```python
from build123d import *

# Parameters (mm, degrees)
F0_R     = 6
F0_R_2   = 4
F1_DEPTH = 1
F2_DEPTH = 7
F3_R     = 6
F3_R_2   = 4
F4_DEPTH = 2
F3_R_3   = 3.9
F3_R_4   = 0.65
F5_DEPTH = 1
F6_SIZE  = 1.5
F7_SIZE  = 0.5


with BuildPart() as f1:
    # F0 (on Top) → F1 (new body)
    with BuildSketch(Plane.XY):
        Circle(F0_R)
        Circle(F0_R_2, mode=Mode.SUBTRACT)
    extrude(amount=F1_DEPTH)

    # F0 (on Top) → F2 (join)
    with BuildSketch(Plane.XY):
        Circle(F0_R_2)
        with BuildLine():
            ThreePointArc((1.1397100223, -2.6552182762), (0.217322658, -3.2453920843), (0.0680019491, -2.1605847745))
            Line((0.0680019491, -2.1605847745), (-2.1226334177, 0.4088743166))
            ThreePointArc((-2.1226334177, 0.4088743166), (-3.1568681461, 1.1210189597), (-1.9051222763, 1.0214009718))
            Line((-1.9051222763, 1.0214009718), (1.415412254, 1.6338173044))
            ThreePointArc((1.415412254, 1.6338173044), (1.9954389417, 2.3990096505), (2.7046314686, 1.7517104579))
            ThreePointArc((2.7046314686, 1.7517104579), (2.4295432969, 1.2207291767), (1.8371203272, 1.1391838027))
            Line((1.8371203272, 1.1391838027), (0.7072211637, -2.0426916209))
            ThreePointArc((0.7072211637, -2.0426916209), (1.0206913035, -2.2803064478), (1.1397100223, -2.6552182762))
        make_face(mode=Mode.SUBTRACT)
        with BuildLine():
            Line((-2.1226334177, 0.4088743166), (0.0680019491, -2.1605847745))
            ThreePointArc((0.0680019491, -2.1605847745), (0.3718168688, -2.0159990615), (0.7072211637, -2.0426916209))
            Line((0.7072211637, -2.0426916209), (1.8371203272, 1.1391838027))
            ThreePointArc((1.8371203272, 1.1391838027), (1.5599979669, 1.3300023847), (1.415412254, 1.6338173044))
            Line((1.415412254, 1.6338173044), (-1.9051222763, 1.0214009718))
            ThreePointArc((-1.9051222763, 1.0214009718), (-1.8970422983, 0.9627003452), (-1.8943414909, 0.9035078183))
            ThreePointArc((-1.8943414909, 0.9035078183), (-1.9541676828, 0.631120454), (-2.1226334177, 0.4088743166))
        make_face()
    extrude(amount=F2_DEPTH)

    # F3 (on face) → F4 (join)
    with BuildSketch(Plane.XY.offset(7)):
        Circle(F3_R)
        Circle(F3_R_2, mode=Mode.SUBTRACT)
    extrude(amount=-F4_DEPTH)

    # F3 (on face) → F5 (cut)
    with BuildSketch(Plane.XY.offset(7)):
        Circle(F3_R_3)
        with Locations((0.4897100223, -2.6552182762)):
            Circle(F3_R_4, mode=Mode.SUBTRACT)
        with Locations((-2.5443414909, 0.9035078183)):
            Circle(F3_R_4, mode=Mode.SUBTRACT)
        with Locations((2.0546314686, 1.7517104579)):
            Circle(F3_R_4, mode=Mode.SUBTRACT)
    extrude(amount=-F5_DEPTH, mode=Mode.SUBTRACT)

    # F6
    f6_edges = [f1.edges().sort_by_distance(p)[0] for p in [
        (-6, 0, 5),
    ]]
    chamfer(f6_edges, length=F6_SIZE)

    # F7
    f7_edges = [f1.edges().sort_by_distance(p)[0] for p in [
        (-6, 0, 1),
    ]]
    chamfer(f7_edges, length=F7_SIZE)


solid = f1.part
```
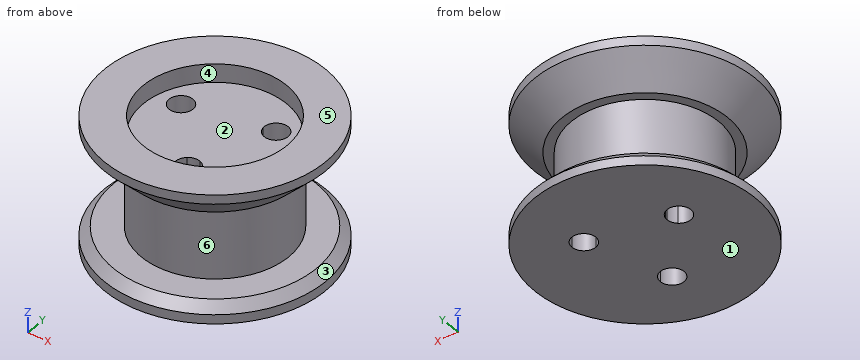
The model under review builds one solid part; all positions refer to its coordinate system, in mm. Face numbers are marked on the shaded views. A direction names the side the tool comes from. Round coordinates to 2 decimals unless told otherwise and drop trailing zeros. Loops run counter-clockwise (first coordinate to the right, second up) from the corner with the lowest first, then second, coordinate; pieces in that order, holes last.
Item 1: Mouldability with a two-part tool opening along X and no side actions: class the marked faces 4, 5 and 6 as released by +X, released by -X, zero draft, split by the parting line, or undercut.
Determined:
face 4: undercut
face 5: zero draft
face 6: split by the parting line
Item 2: Take a section at C-C (z = 3.5). Write out the cut boundary in (x, y).
Determined:
outline: circle Ø8 at (0, 0); hole circle Ø1.3 at (-2.54, 0.9); hole circle Ø1.3 at (0.49, -2.66); hole circle Ø1.3 at (2.05, 1.75)
Item 3: Take a section at B-B (y = 0). Write out the cut boundary in (x, z).
Determined:
outline: (-6, 0) - (6, 0) - (6, 0.5) - (5.5, 1) - (4, 1) - (4, 5) - (4.5, 5) - (6, 6.5) - (6, 7) - (3.9, 7) - (3.9, 6) - (-3.9, 6) - (-3.9, 7) - (-6, 7) - (-6, 6.5) - (-4.5, 5) - (-4, 5) - (-4, 1) - (-5.5, 1) - (-6, 0.5) - close
Item 4: Take a section at A-A (z = 5.25). Write out the cut boundary in (x, y), then the cut area to 3 significant figures.
Determined:
outline: circle Ø9.5 at (0, 0); hole circle Ø1.3 at (-2.54, 0.9); hole circle Ø1.3 at (0.49, -2.66); hole circle Ø1.3 at (2.05, 1.75)
area: 66.9 mm2
Item 5: For the marked faces 1, 2 and 3, list the 3-axis set-ups (+Z, -Z, +X, -X, +Y, -Y) from which the entire face can be reached by the end or side of a thin tool; tool diameter is ignored.
Determined:
face 1: -Z, +X, -X, +Y, -Y
face 2: +Z
face 3: none
Item 6: For line 1 (Z direction, x = -4, y = 3); line 2 (Z direction, x = 3, y = 3); line 3 (X direction, y = -2.5, z = 1.5), list the stretches that pass through material, from the lowest coordinate up.
Determined:
line 1: z = 0 to 1, 5.5 to 7
line 2: z = 0 to 1, 5 to 7
line 3: x = -3.12 to -0.14, 1.12 to 3.12
Item 7: Clearance check with flat-ended pins moving along their axes: pin 1 Ø2 at (x, z) = (-3.5, 5) entering from -Y; pin 2 Ø1.5 at (x, y) = (-2.54, 0.9) entering from +Z. State where each tip first meets the part, or that it passes through.
Determined:
pin 1: stops at y = -4.45
pin 2: stops at z = 6
